Work out the finished part from the listing and answer in its coordinate system (mm). Coordinates: 2 decimals unless noted, no trailing zeros. Write each loop counter-clockwise with the first axis right and the second up, starting at its lowest first coordinate (ties: lowest second). Pieces come first, ordered by that corner, then holes. Notation, with made-up numbers: (-26.5, 28) - (31.5, 28) arc R9 cw to (31.5, 33) - close; hole circle Ø5 at (9.5, 12.25). An arc over 180 degrees is marked (long way). Use one line per item in the form item = value. Start each with the question number.
Item 1: A cutting plane is placed at A-A (z = 125). Write down the section's boundary in (x, y), then the cut area to 3 significant figures.
Item 2: A cutting plane is placed at B-B (x = -6.25). Write down the section's boundary in (y, z).
Item 3: A cutting plane is placed at D-D (z = 189). Write down the section's boundary in (x, y).
Item 4: Consider probe 1 along X at (y, z) = (-4.7, 77); probe 2 along Y at (x, z) = (-6.5, 104.5); probe 3 along X at (y, z) = (-0.75, 104). Determine where each line is inside the solid, lowest interval first.
Item 5: A cutting plane is placed at C-C (y = 0). Give the number of separate pieces and of enclosed holes in the cut face, then the cut area to 3 significant figures.
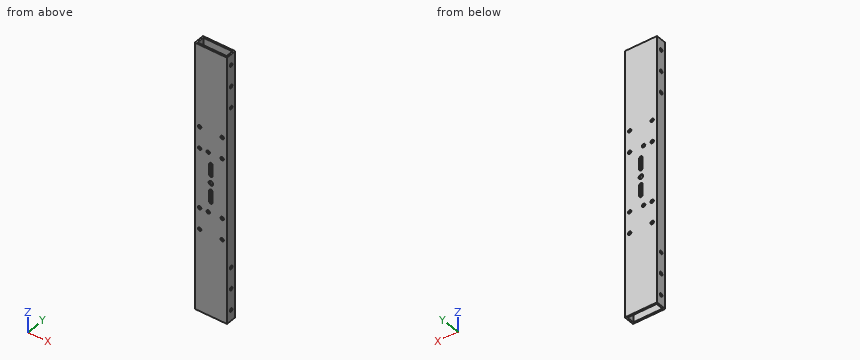
from build123d import *

# Parameters (mm, degrees)
SKETCH_1_W          = 30
SKETCH_1_H          = 10
SKETCH_1_W_2        = 27
SKETCH_1_H_2        = 7
EXTRUDE_1_DEPTH     = 250
SKETCH_2_R          = 1.6
CUT_EXTRUDE_1_DEPTH = 252.843205189
SKETCH_3_R          = 1.6
CUT_EXTRUDE_2_DEPTH = 251.64915719
SKETCH_4_R          = 2.15
CUT_EXTRUDE_3_DEPTH = 251.64915719


with BuildPart() as part:
    # 草图1 → 凸台-拉伸1 (new body)
    with BuildSketch(Plane.XY):
        Rectangle(SKETCH_1_W, SKETCH_1_H)
        Rectangle(SKETCH_1_W_2, SKETCH_1_H_2, mode=Mode.SUBTRACT)
    extrude(amount=EXTRUDE_1_DEPTH)

    # 草图2 → 切除-拉伸1 (cut, through all)
    with BuildSketch(Plane(origin=(15, 0, 0), x_dir=(0, 0, -1), z_dir=(1, 0, 0))):
        with Locations((-240, 0)):
            Circle(SKETCH_2_R)
        with Locations((-220, 0)):
            Circle(SKETCH_2_R)
        with Locations((-200, 0)):
            Circle(SKETCH_2_R)
        with Locations((-50, 0)):
            Circle(SKETCH_2_R)
        with Locations((-30, 0)):
            Circle(SKETCH_2_R)
        with Locations((-10, 0)):
            Circle(SKETCH_2_R)
    extrude(amount=-CUT_EXTRUDE_1_DEPTH, mode=Mode.SUBTRACT)

    # 草图3 → 切除-拉伸2 (cut, through all)
    with BuildSketch(Plane(origin=(0, 5, 0), x_dir=(1, 0, 0), z_dir=(0, 1, 0))):
        with Locations(Location((-2.5, -97, 0), (0, 0, 270))):
            Circle(SKETCH_3_R)
        with Locations(Location((10.5, -97, 0), (0, 0, 270))):
            Circle(SKETCH_3_R)
        with Locations(Location((-2.5, -153, 0), (0, 0, 270))):
            Circle(SKETCH_3_R)
        with Locations(Location((10.5, -153, 0), (0, 0, 270))):
            Circle(SKETCH_3_R)
        with Locations(Location((10.5, -173, 0), (0, 0, 270))):
            Circle(SKETCH_3_R)
        with Locations(Location((10.5, -77, 0), (0, 0, 270))):
            Circle(SKETCH_3_R)
        with Locations(Location((-10.5, -173, 0), (0, 0, 270))):
            Circle(SKETCH_3_R)
        with Locations(Location((-10.5, -153, 0), (0, 0, 270))):
            Circle(SKETCH_3_R)
        with Locations(Location((-10.5, -77, 0), (0, 0, 270))):
            Circle(SKETCH_3_R)
        with Locations(Location((-10.5, -97, 0), (0, 0, 270))):
            Circle(SKETCH_3_R)
    extrude(amount=-CUT_EXTRUDE_2_DEPTH, mode=Mode.SUBTRACT)

    # 草图4 → 切除-拉伸3 (cut, through all)
    with BuildSketch(Plane(origin=(0, 5, 0), x_dir=(1, 0, 0), z_dir=(0, 1, 0))):
        with Locations(Location((0, -125, 0), (0, 0, 270))):
            Circle(SKETCH_4_R)
        with BuildLine():
            Line((-1.65, -107.5), (-1.65, -117.5))
            ThreePointArc((-1.65, -117.5), (0, -119.15), (1.65, -117.5))
            Line((1.65, -117.5), (1.65, -107.5))
            ThreePointArc((1.65, -107.5), (0, -105.85), (-1.65, -107.5))
        make_face()
        with BuildLine():
            Line((1.65, -142.5), (1.65, -132.5))
            ThreePointArc((1.65, -132.5), (0, -130.85), (-1.65, -132.5))
            Line((-1.65, -132.5), (-1.65, -142.5))
            ThreePointArc((-1.65, -142.5), (0, -144.15), (1.65, -142.5))
        make_face()
    extrude(amount=-CUT_EXTRUDE_3_DEPTH, mode=Mode.SUBTRACT)


solid = part.part
Answer:
q1.outline = (-15, -5) - (-2.15, -5) - (-2.15, -3.5) - (-13.5, -3.5) - (-13.5, 3.5) - (-2.15, 3.5) - (-2.15, 5) - (-15, 5) - close; (2.15, -5) - (15, -5) - (15, 5) - (2.15, 5) - (2.15, 3.5) - (13.5, 3.5) - (13.5, -3.5) - (2.15, -3.5) - close
q1.area = 98.1 mm²
q2.outline = (-5, 0) - (-3.5, 0) - (-3.5, 250) - (-5, 250) - close; (3.5, 0) - (5, 0) - (5, 250) - (3.5, 250) - close
q3.outline = (-15, -5) - (15, -5) - (15, 5) - (-15, 5) - close; hole (-13.5, -3.5) - (13.5, -3.5) - (13.5, 3.5) - (-13.5, 3.5) - close
q4.probe_1 = -15 to -12.1, -8.9 to 8.9, 12.1 to 15
q4.probe_2 = -5 to -3.5, 3.5 to 5
q4.probe_3 = -15 to -13.5, 13.5 to 15
q5.separate_pieces = 14
q5.enclosed_holes = 0
q5.area = 692 mm²
